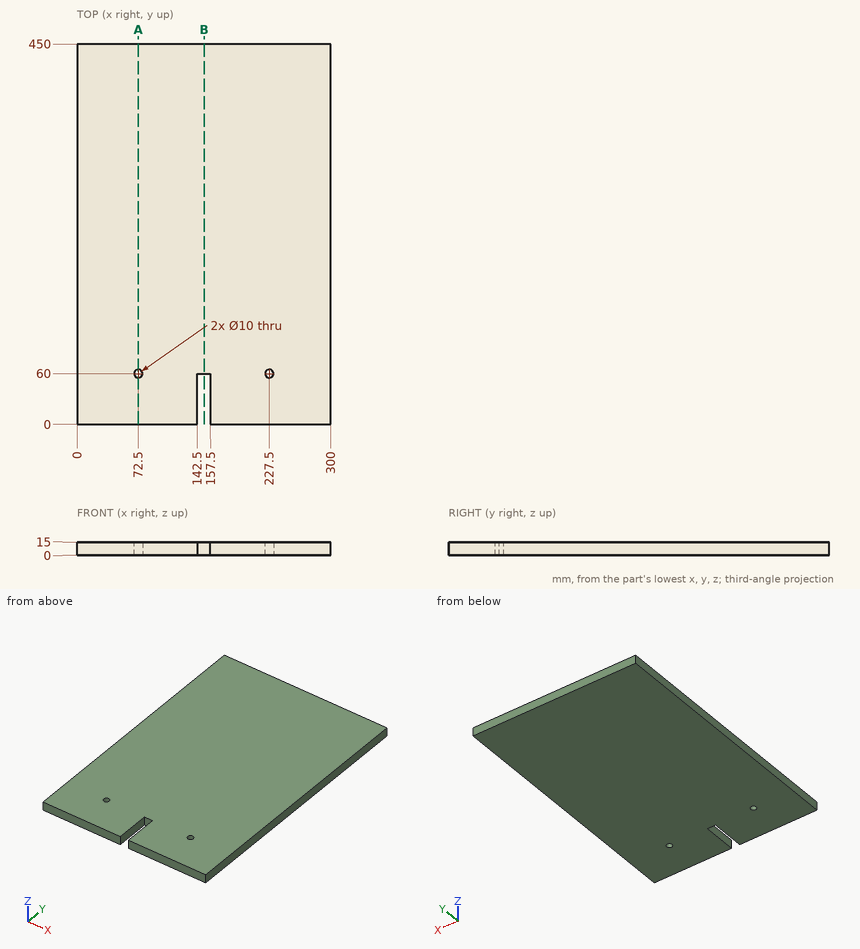
Design review of the part shown in the three views and the two pictorial views. Dimensions are in mm from the part's minimum x, y and z. Give positions to 0.01 mm unless a question says otherwise; leave off trailing zeros. Write each loop counter-clockwise with the first axis right and the second up, starting at its lowest first coordinate (ties: lowest second). Pieces come first, ordered by that corner, then holes. Notation, with made-up numbers: (84, 45.5) - (90, 45.5) arc R8 ccw to (90, 49.5) - close; hole circle Ø7 at (40.25, 23). An arc over 180 degrees is marked (long way). Return JSON: item names as keys, results as strings. Group by question number.
(1) To check wall thickness, follow probe 1 along Y at (x, z) = (72.5, 12); probe 2 along Y at (x, z) = (156.5, 13.5). State the ranges of each line that lie inside material, in increasing order.
(2) Insertion check: pin 1 (1 mm diameter, centred on x = 85, y = 225, fed in from -Z); pin 2 (7.5 mm diameter, centred on x = 151, z = 10, fed in from -Y); pin 3 (9 mm diameter, centred on x = 72.5, y = 60, fed in from -Z). Each pin has a flat end and moves straight along its axis. Give the tip position at first contact, or say it passes through.
(3) We need section A-A, the plane x = 72.5. Give the boundary of the cut face in (y, z), then the cut area to 3 significant figures.
(4) We need section B-B, the plane x = 150.5. Give the boundary of the cut face in (y, z), then the cut area to 3 significant figures.
Reported:
{
 "1": {"probe 1": "y = 0 to 55, 65 to 450", "probe 2": "y = 60 to 450"},
 "2": {"pin 1": "stops at z = 0", "pin 2": "stops at y = 60", "pin 3": "passes through"},
 "3": {"outline": "(0, 0) - (55, 0) - (55, 15) - (0, 15) - close; (65, 0) - (450, 0) - (450, 15) - (65, 15) - close", "area": "6,600 mm2"},
 "4": {"outline": "(60, 0) - (450, 0) - (450, 15) - (60, 15) - close", "area": "5,850 mm2"}
}
